Input: dimensioned drawing with shaded views. Units: mm. Origin: part minimum x, y, z. A direction names the side the tool comes from. Give positions to 0.01 mm unless a question says otherwise; leave off trailing zeros. Write each loop counter-clockwise with the first axis right and the second up, starting at its lowest first coordinate (ties: lowest second). Pieces come first, ordered by that corner, then holes. Notation, with made-up numbers: (89.5, 0.25) -> (145.5, 0.25) arc R20 cw to (145.5, 29.25) -> close; hole circle Ø9 at (40.5, 88.25). An arc over 180 degrees is marked (long way). Answer as a JSON object with one key per item and string values.
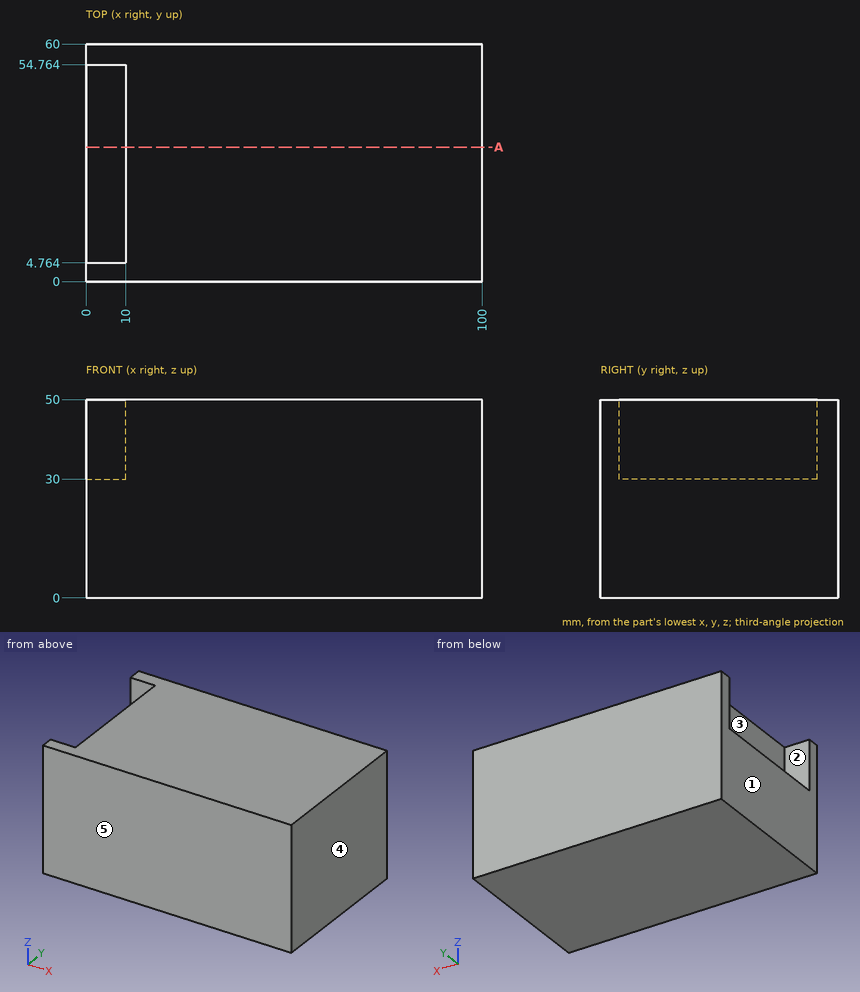
Q1. Mould query, pull axis X, two halves, no side actions, for the marked faces 3, 4 and 5. Classes: pulls with the +X half, pulls with the -X half, needs draft (parallel to the pull), parting line crosses it, or undercut.
Values:
{"face 3": "pulls with the -X half", "face 4": "pulls with the +X half", "face 5": "needs draft"}
Q2. Cut plane A-A (y = 34). Return the cut outline in (x, z).
Values:
{"outline": "(0, 0) -> (100, 0) -> (100, 50) -> (10, 50) -> (10, 30) -> (0, 30) -> close"}
Q3. First-contact query: P1, Ø4, axis at y = 44, z = 40.5, coming from the -X side; P2, Ø5, axis at x = 6, y = 25.5, coming from the +Z side. Flat tips, straight axial feed; report the tip coordinate or a pass-through.
Values:
{"P1": "x = 10", "P2": "z = 30"}
Q4. Material intervals for L1, parallel to X at y = 54, z = 40, sorted ascending. Write a range as from..to.
Values:
{"L1": "10..100"}
Q5. Set-up query: the marked faces 1 and 2. Return all of +Z, -Z, +X, -X, +Y, -Y with unobstructed straight access to the full face (end or side cutting, diameter ignored); none if empty.
Values:
{"face 1": "+Z, -Z, -X, +Y, -Y", "face 2": "+Z, -X"}
